Work out the finished part from the listing and answer in its coordinate system (mm). A direction names the side the tool comes from. Coordinates: 2 decimals unless noted, no trailing zeros. Write each loop counter-clockwise with the first axis right and the second up, starting at its lowest first coordinate (ties: lowest second). Pieces come first, ordered by that corner, then holes. Notation, with made-up numbers: M -9,34 L 49,34 A17 ccw 49,38 Z; hole C 11.5,-37.5 d9. An arc over 180 degrees is marked long. Answer as CSV lines item,"result". Start each with the question number.
(1) A cutting plane is placed at A-A on x = 12. Give the vertices of the cut face in (y, z).
(2) Find the intervals of material crossed by L1, parallel to Z at x = 18.5, y = -13; L2, parallel to Z at x = 64, y = -7; L3, parallel to X at y = -14, z = -48, in increasing order. Write a range as [from, to].
(3) For faces 1 (the flat face through (7.195, -8, -48)), 2 (the flat face through (-24, -8, -54.107)), 3 (the flat face through (40.005, -8, -60)), determine the directions among +Z, -Z, +X, -X, +Y, -Y from which every point of the face is accessible in a straight line to the end or side of a thin tool.
(4) A cutting plane is placed at C-C on x = 59.5. Give the vertices of the cut face in (y, z), then the cut area to 3 significant figures.
(5) The mould has two halves that part along Z. Classify faces 4 (the flat face through (-1, 0.254, -59)), 5 (the flat face through (-1, -8, -65.62)), 6 (the flat face through (-49, -8, -42.307)): released by +Z, released by -Z, zero draft, split by the parting line, or undercut.
(6) A cutting plane is placed at B-B on y = -3.5. Give the vertices of the cut face in (x, z) (3 decimals), then the cut area to 3 significant figures.
(7) Flat-ended cylindrical pins translate along their axes: P1, Ø3.5, axis at y = -6, z = -45.5, coming from the +X side; P2, Ø8, axis at x = -14.5, z = -40.5, coming from the +Y side; P3, Ø3.5, axis at y = -4.5, z = -47.5, coming from the -X side. Find the tip coordinate at first contact, or state that the pin passes through.
from build123d import *

# Parameters (mm, degrees)
F0_W     = 176.3164922595
F0_H     = 107.0637442172
F0_W_2   = 167.9538153112
F0_H_2   = 100.156404078
F1_DEPTH = 16.002
F2_W     = 14.965901617
F2_H     = 11.8000358343
F2_W_2   = 112.8198541701
F2_H_2   = 94.6880914271
F3_DEPTH = 16.256


with BuildPart() as f1:
    # F0 (on Front) → F1 (new body)
    with BuildSketch(Plane.XZ):
        with Locations((-1.561973244, 11.2244244665)):
            Rectangle(F0_W, F0_H)
        with Locations((-1.1848155409, 10.9366178513)):
            Rectangle(F0_W_2, F0_H_2, mode=Mode.SUBTRACT)
        with Locations((-1.1848155409, 10.9366178513)):
            Rectangle(F0_W_2, F0_H_2)
    extrude(amount=F1_DEPTH)

    # F2 (on face) → F3 (join)
    with BuildSketch(Plane.XZ.offset(16.002)):
        Polygon((7.1951453574, -54.1074834764), (-7.7707562596, -54.1074834764), (-40.0050021708, -54.1074834764), (-40.0050021708, -65.6197145581), (40.0049984455, -65.6197145581), (40.0049984455, -54.1074834764), align=None)
        with Locations((-0.2878054511, -48.2074655592)):
            Rectangle(F2_W, F2_H)
        with Locations((0.2878028899, 11.3683287054)):
            Rectangle(F2_W_2, F2_H_2)
    extrude(amount=-F3_DEPTH)


solid = f1.part
Here are the results:
1,outline,"M -16,-65.62 L 0.25,-65.62 L 0.25,-54.11 L -16,-54.11 Z; M -16,-42.31 L 0,-42.31 L 0,-35.98 L 0.25,-35.98 L 0.25,58.71 L 0,58.71 L 0,64.76 L -16,64.76 Z"
2,L1,"z = [-65.62, -54.11], [-42.31, 64.76]"
2,L2,"z = [-42.31, 64.76]"
2,L3,"x = [-7.77, 7.2]"
3,face 1,"+X, +Y, -Y"
3,face 2,"-X, +Y, -Y"
3,face 3,"-Z, +X, +Y, -Y"
4,outline,"M -16,-42.31 L 0,-42.31 L 0,64.76 L -16,64.76 Z"
4,area,"1,710 mm^2"
5,face 4,"zero draft"
5,face 5,"released by -Z"
5,face 6,"undercut"
6,outline,"M -89.72,-42.307 L -7.771,-42.307 L -7.771,-54.107 L -40.005,-54.107 L -40.005,-65.62 L 40.005,-65.62 L 40.005,-54.107 L 7.195,-54.107 L 7.195,-42.307 L 86.596,-42.307 L 86.596,64.756 L -89.72,64.756 Z"
6,area,"20,000 mm^2"
7,P1,"stops at x = 7.2"
7,P2,"stops at y = 0"
7,P3,"stops at x = -7.77"
